from build123d import *

# Parameters (mm, degrees)
ESQUISSE1_R                = 175
BOSS_EXTRU_1_DEPTH         = 5
ESQUISSE2_W                = 18
ESQUISSE2_H                = 5
ESQUISSE2_W_2              = 5
ESQUISSE2_H_2              = 20
ESQUISSE2_H_3              = 10
ESQUISSE2_H_4              = 15
ESQUISSE2_H_5              = 15.5
ESQUISSE2_W_3              = 20
ESQUISSE2_H_6              = 6.5
ENL_V_MAT_EXTRU_1_DEPTH    = 5
ESQUISSE6_R                = 12.5
ESQUISSE6_W                = 50
ESQUISSE6_H                = 50
ENL_V_MAT_EXTRU_6_DEPTH    = 5
TROUS_DE_CENTRAGE_4_0MM1_D = 4


with BuildPart() as part:
    # Esquisse1 → Boss.-Extru.1 (new body)
    with BuildSketch(Plane.XY):
        with Locations((148.080426897, -12.110171348)):
            Circle(ESQUISSE1_R)
    extrude(amount=BOSS_EXTRU_1_DEPTH)

    # Esquisse2 → Enlèv. mat.-Extru.1 (cut)
    with BuildSketch(Plane.XY.offset(5)):
        Polygon((135.311788567, 53.777441362), (135.311788567, 48.777441362), (145.311788567, 48.777441362), (145.311788567, 42.277441362), (150.311788567, 42.277441362), (150.311788567, 48.777441362), (155.311788567, 48.777441362), (155.311788567, 53.777441362), align=None)
        with Locations((14, 69.777441362)):
            Rectangle(ESQUISSE2_W, ESQUISSE2_H)
        with Locations((-2.5, 52.277441362)):
            Rectangle(ESQUISSE2_W_2, ESQUISSE2_H_2)
        with Locations((-2.5, 9.277441362)):
            Rectangle(ESQUISSE2_W_2, ESQUISSE2_H_2)
        with Locations((14, -8.222558638)):
            Rectangle(ESQUISSE2_W, ESQUISSE2_H)
        with Locations((29.5, 9.277441362)):
            Rectangle(ESQUISSE2_W_2, ESQUISSE2_H_3)
        with Locations((29.5, 30.777441362)):
            Rectangle(ESQUISSE2_W_2, ESQUISSE2_H_4)
        with Locations((29.5, 52.277441362)):
            Rectangle(ESQUISSE2_W_2, ESQUISSE2_H_3)
        with Locations((57.36, 41.027441362)):
            Rectangle(ESQUISSE2_W_2, ESQUISSE2_H_5)
        with Locations((57.36, 20.527441362)):
            Rectangle(ESQUISSE2_W_2, ESQUISSE2_H_5)
        with Locations((95.311788567, 51.277441362)):
            Rectangle(ESQUISSE2_W_3, ESQUISSE2_H)
        with Locations((147.811788567, 34.027441362)):
            Rectangle(ESQUISSE2_W_2, ESQUISSE2_H_6)
        Polygon((292.702456717, 69.607306773), (283.702456717, 54.018849505), (279.372329698, 56.518849505), (288.372329698, 72.107306773), align=None)
        Polygon((289.042202679, 83.267560811), (286.542202679, 78.937433792), (269.221694603, 88.937433792), (271.721694603, 93.267560811), align=None)
        Polygon((251.803110316, 104.767560811), (249.303110316, 100.437433792), (231.982602241, 110.437433792), (234.482602241, 114.767560811), align=None)
        Polygon((225.152475222, 108.607306773), (216.152475222, 93.018849505), (211.822348203, 95.518849505), (220.822348203, 111.107306773), align=None)
        Polygon((231.472983297, 79.55474789), (228.972983297, 75.224620871), (220.31272926, 80.224620871), (222.81272926, 84.55474789), align=None)
        Polygon((252.257592988, 67.55474789), (249.757592988, 63.224620871), (236.767211932, 70.724620871), (239.267211932, 75.05474789), align=None)
        Polygon((268.71207566, 58.05474789), (266.21207566, 53.724620871), (257.551821622, 58.724620871), (260.051821622, 63.05474789), align=None)
        Polygon((247.420859728, 38.17728014), (244.920859728, 33.847153121), (231.497465969, 41.597153121), (233.997465969, 45.92728014), align=None)
        Polygon((229.66733895, 48.42728014), (227.16733895, 44.097153121), (213.743945192, 51.847153121), (216.243945192, 56.17728014), align=None)
        Polygon((211.525092463, -33.996012539), (207.194965444, -31.496012539), (202.194965444, -40.156266577), (196.56580032, -36.906266577), (194.06580032, -41.236393596), (199.694965444, -44.486393596), (197.194965444, -48.816520615), (201.525092463, -51.316520615), align=None)
        Polygon((236.525092463, 9.30525765), (226.525092463, -8.015250425), (222.194965444, -5.515250425), (232.194965444, 11.80525765), align=None)
        Polygon((192.235673301, -34.406266577), (189.735673301, -38.736393596), (184.106508176, -35.486393596), (186.606508176, -31.156266577), align=None)
        Polygon((146.538823973, -178.215262181), (137.538823973, -162.626804912), (141.868950992, -160.126804912), (150.868950992, -175.715262181), align=None)
        Polygon((160.199078011, -181.875516218), (157.699078011, -177.545389199), (175.019586086, -167.545389199), (177.519586086, -171.875516218), align=None)
        Polygon((197.438170373, -160.375516218), (194.938170373, -156.045389199), (212.258678449, -146.045389199), (214.758678449, -150.375516218), align=None)
        Polygon((214.088805468, -139.215262181), (205.088805468, -123.626804912), (209.418932487, -121.126804912), (218.418932487, -136.715262181), align=None)
        Polygon((185.768297392, -130.162703297), (183.268297392, -125.832576278), (191.92855143, -120.832576278), (194.42855143, -125.162703297), align=None)
        Polygon((164.983687701, -142.162703297), (162.483687701, -137.832576278), (175.474068758, -130.332576278), (177.974068758, -134.662703297), align=None)
        Polygon((148.52920503, -151.662703297), (146.02920503, -147.332576278), (154.689459067, -142.332576278), (157.189459067, -146.662703297), align=None)
        Polygon((141.960420962, -123.285235548), (139.460420962, -118.955108529), (152.88381472, -111.205108529), (155.38381472, -115.535235548), align=None)
        Polygon((159.713941739, -113.035235548), (157.213941739, -108.705108529), (170.637335498, -100.955108529), (173.137335498, -105.285235548), align=None)
        Polygon((97.404399659, -56.111942869), (101.734526678, -53.611942869), (96.734526678, -44.951688831), (102.363691803, -41.701688831), (99.863691803, -37.371561812), (94.234526678, -40.621561812), (91.734526678, -36.291434793), (87.404399659, -38.791434793), align=None)
        Polygon((122.404399659, -99.413213058), (112.404399659, -82.092704982), (116.734526678, -79.592704982), (126.734526678, -96.913213058), align=None)
        Polygon((106.693818822, -39.201688831), (104.193818822, -34.871561812), (109.822983946, -31.621561812), (112.322983946, -35.951688831), align=None)
    extrude(amount=-ENL_V_MAT_EXTRU_1_DEPTH, mode=Mode.SUBTRACT)

    # Esquisse6 → Enlèv. mat.-Extru.6 (cut)
    with BuildSketch(Plane.XY.offset(5)):
        with Locations((173.06, 32.277441362)):
            Circle(ESQUISSE6_R)
        with Locations((174.031440566, -55.936922587)):
            Circle(ESQUISSE6_R)
        with Locations((97.149840124, -12.67103282)):
            Circle(ESQUISSE6_R)
        with Locations((148.080426897, -12.110171348)):
            Rectangle(ESQUISSE6_W, ESQUISSE6_H)
    extrude(amount=-ENL_V_MAT_EXTRU_6_DEPTH, mode=Mode.SUBTRACT)

    # Trous de centrage Ø4.0mm1 (through all)
    with Locations(Plane(origin=(148.080426897, -12.110171348, -78), x_dir=(1, 0, 0), z_dir=(0, 0, -1))):
        with Locations((65.70121345, -88.022614393), (117.662737677, -58.022614393), (-109.080426897, -72.887612711), (-109.080426897, -12.887612711), (-8.58231078, 130.910227103), (43.379213447, 100.910227103)):
            Hole(TROUS_DE_CENTRAGE_4_0MM1_D / 2)


solid = part.part
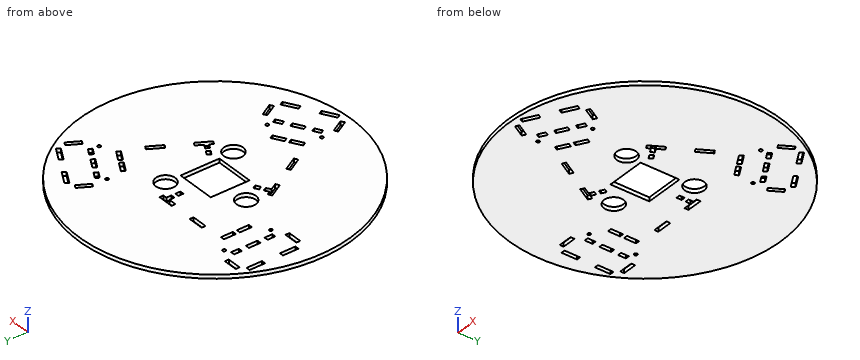
Here's how the part is built. I have some questions about the finished solid (model axes, mm). Coordinates: 2 decimals unless noted, no trailing zeros. Order: outer loops, then holes, each group sorted by start corner. A loop starts at its lowest first (then second) coordinate and runs counter-clockwise, first axis right, second up. Notation, with made-up numbers: M -10,31.5 L 7,31.5 A21 cw 7,39.5 Z; hole C -15.5,65.25 d8. An arc over 180 degrees is marked long. Answer as CSV lines item,"result". Start each with the question number.
1. For pin 1 (2.5 mm diameter, centred on y = 34.5, z = 3, fed in from +X); pin 2 (5 mm diameter, centred on x = 139.5, y = -143.02, fed in from +Z); pin 3 (1.5 mm diameter, centred on x = 145, z = 2, fed in from +Y); pin 4 (2.5 mm diameter, centred on x = 100.5, z = 2.5, fed in from +Y), each with a flat end and sliding along its axis, tell me the tip position at first contact or that it passes through.
2. I want a section at A-A, the plane z = 2.4. Count the separate pieces of the cut face and the enclosed holes in it, and give its area (3 significant figures).
3. I need wall thicknesses on line 1 (Y direction, x = 216.5, z = 3.4); line 2 (X direction, y = 65, z = 0.3); line 3 (Y direction, x = 12, z = 3.25). Which ranges of each line are inside material? Lowest first, please. Write a range as [from, to].
4. I want a section at B-B, the plane x = 46. Write out the boundary of the cut face in (y, z).
Recorded:
1,pin 1,"stops at x = 317.1"
1,pin 2,"stops at z = 5"
1,pin 3,"stops at y = 162.87"
1,pin 4,"stops at y = 156.65"
2,separate pieces,"1"
2,enclosed holes,"46"
2,area,"89,200 mm2"
3,line 1,"y = [-173.18, -137.82], [-133.39, 50.26], [56.03, 93.62], [103.62, 148.96]"
3,line 2,"x = [-9.02, 246.68], [250.78, 284.27], [290.04, 305.18]"
3,line 3,"y = [-122.14, -10.72], [-5.72, 67.28], [72.28, 97.92]"
4,outline,"M -154.25,0 L 130.03,0 L 130.03,5 L -154.25,5 Z"
